from build123d import *

# Parameters (mm, degrees)
F1_DEPTH = 4
F3_D     = 1.89
F5_D     = 1.89


with BuildPart() as f1:
    # F0 (on Top) → F1 (new body)
    with BuildSketch(Plane.XY):
        with BuildLine():
            ThreePointArc((0, 3), (0.8786796564, 0.8786796564), (3, 0))
            Line((3, 0), (32, 0))
            ThreePointArc((32, 0), (34.1213203436, 0.8786796564), (35, 3))
            ThreePointArc((35, 3), (34.1213203436, 5.1213203436), (32, 6))
            Line((32, 6), (3, 6))
            ThreePointArc((3, 6), (0.8786796564, 5.1213203436), (0, 3))
        make_face()
    extrude(amount=F1_DEPTH)

    # F3 (through all)
    with Locations(Plane.XY.offset(4)):
        with Locations((3, 3)):
            Hole(F3_D / 2)

    # F5 (through all)
    with Locations(Plane(origin=(0, 0, 0), x_dir=(1, 0, 0), z_dir=(0, 0, -1))):
        with Locations((32.3587208986, -2.8431627434)):
            Hole(F5_D / 2)


solid = f1.part
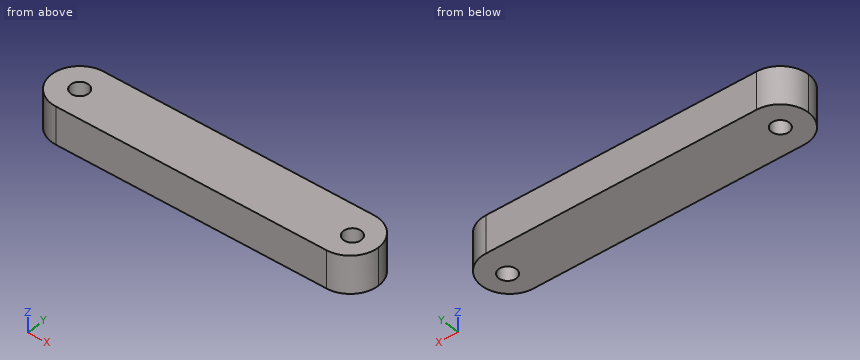
Input: part model. Units: mm. Frame: model coordinates. Round coordinates to 2 decimals unless told otherwise and drop trailing zeros. Loops run counter-clockwise (first coordinate to the right, second up) from the corner with the lowest first, then second, coordinate; pieces in that order, holes last. Notation, with made-up numbers: (19, 43.5) -> (73, 43.5) arc R20 ccw to (73, 53.5) -> close; hole circle Ø4 at (72.25, -39.5). An arc over 180 degrees is marked (long way). Answer as a JSON object with one key per item and string values. Group by question number.
1) Section query C-C on y = 0.5. Output: boundary loops of the cut face in (x, z).
2) Section query B-B on z = 0.6. Output: boundary loops of the cut face in (x, y) (3 decimals).
3) Pin query (flat end, axial travel): pin 1 (1.5 mm diameter, centred on y = 4, z = 0.5, fed in from -X). Return the tip coordinate at first contact, or that it passes through.
4) Ray query, L1, parallel to X at y = 2.5, z = 2.65; L2, parallel to Y at x = 3, z = 1.45 (3 decimals); L3, parallel to Y at x = 32, z = 1.6. Return the intervals inside material, ascending.
5) Section query D-D on y = 5.25. Output: boundary loops of the cut face in (x, z).
6) Section query A-A on y = 2.5. Output: boundary loops of the cut face in (x, z).
Reply:
{
 "1": {"outline": "(1.34, 0) -> (33.66, 0) -> (33.66, 4) -> (1.34, 4) -> close"},
 "2": {"outline": "(3, 0) -> (32, 0) arc R3 ccw to (32, 6) -> (3, 6) arc R3 ccw to start; hole circle Ø1.89 at (3, 3); hole circle Ø1.89 at (32.359, 2.843)"},
 "3": {"pin 1": "stops at x = 0.01"},
 "4": {"L1": "x = 0.04 to 2.2, 3.8 to 31.48, 33.24 to 34.96", "L2": "y = 0 to 2.055, 3.945 to 6", "L3": "y = 0 to 1.97, 3.72 to 6"},
 "5": {"outline": "(1.02, 0) -> (33.98, 0) -> (33.98, 4) -> (1.02, 4) -> close"},
 "6": {"outline": "(0.04, 0) -> (2.2, 0) -> (2.2, 4) -> (0.04, 4) -> close; (3.8, 0) -> (31.48, 0) -> (31.48, 4) -> (3.8, 4) -> close; (33.24, 0) -> (34.96, 0) -> (34.96, 4) -> (33.24, 4) -> close"}
}
